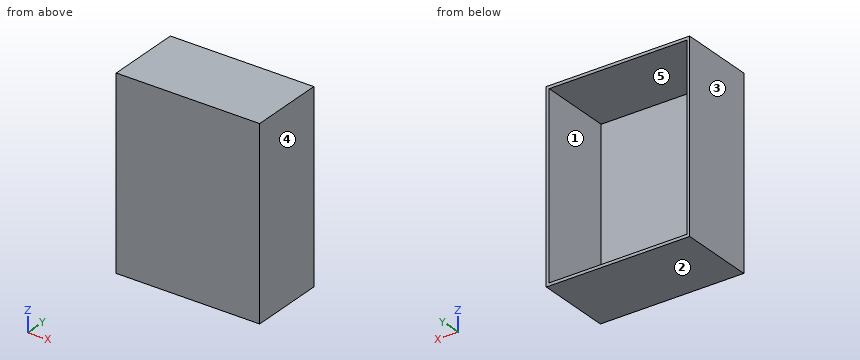
```python
from build123d import *

# Parameters (mm, degrees)
SKETCH2_W   = 99
SKETCH2_H   = 129
SKETCH2_W_2 = 95
SKETCH2_H_2 = 125
WALLS_DEPTH = 50
SKETCH3_W   = 99
SKETCH3_H   = 129
BASE_DEPTH  = 2


with BuildPart() as part:
    # Sketch2 → Walls (new body)
    with BuildSketch(Plane(origin=(0, 0, 0), x_dir=(1, 0, 0), z_dir=(0, 1, 0))):
        Rectangle(SKETCH2_W, SKETCH2_H)
        Rectangle(SKETCH2_W_2, SKETCH2_H_2, mode=Mode.SUBTRACT)
    extrude(amount=WALLS_DEPTH)

    # Sketch3 → Base (add)
    with BuildSketch(Plane.XZ):
        Rectangle(SKETCH3_W, SKETCH3_H)
    extrude(amount=BASE_DEPTH)


solid = part.part
```
The listing builds one solid part. Answer for the finished solid, in the listing's coordinates (mm). Face numbers are marked on the shaded views. A direction names the side the tool comes from. Round coordinates to 2 decimals unless told otherwise and drop trailing zeros. Loops run counter-clockwise (first coordinate to the right, second up) from the corner with the lowest first, then second, coordinate; pieces in that order, holes last. Notation, with made-up numbers: (-8.75, 22.5) - (39.25, 22.5) arc R18 cw to (39.25, 32.5) - close; hole circle Ø4 at (-40, 60.5). An arc over 180 degrees is marked (long way). Return JSON: item names as keys, results as strings. Group by question number.
1. Consider probe 1 along Z at (x, y) = (-37.5, 22); probe 2 along X at (y, z) = (44, -11); probe 3 along Y at (x, z) = (-17, 15). Determine where each line is inside the solid, lowest interval first.
2. The mould has two halves that part along Z. Classify the marked faces 1, 2 and 3: pulls with the +Z half, pulls with the -Z half, needs draft (parallel to the pull), parting line crosses it, or undercut.
3. The part is cut by section C-C on z = 23.5. Determine the outline of the cut face in (x, y).
4. The part is cut by section B-B on x = -19.5. Determine the outline of the cut face in (y, z).
5. The part is cut by section A-A on y = 42. Determine the outline of the cut face in (x, z), then the cut area to 3 significant figures.
6. This flat-tipped pin is pushed along its axis until it touches: P1, Ø10, axis at x = 10, z = 36.5, coming from the +Y side. Where does it stop, or does it pass through?
7. Which of the six approach directions +Z, -Z, +X, -X, +Y, -Y give full straight-line access (tool end or side, diameter ignored) to the marked faces 4 and 5?
Resolved:
{
 "1": {"probe 1": "z = -64.5 to -62.5, 62.5 to 64.5", "probe 2": "x = -49.5 to -47.5, 47.5 to 49.5", "probe 3": "y = -2 to 0"},
 "2": {"face 1": "undercut", "face 2": "pulls with the -Z half", "face 3": "needs draft"},
 "3": {"outline": "(-49.5, -2) - (49.5, -2) - (49.5, 50) - (47.5, 50) - (47.5, 0) - (-47.5, 0) - (-47.5, 50) - (-49.5, 50) - close"},
 "4": {"outline": "(-2, -64.5) - (50, -64.5) - (50, -62.5) - (0, -62.5) - (0, 62.5) - (50, 62.5) - (50, 64.5) - (-2, 64.5) - close"},
 "5": {"outline": "(-49.5, -64.5) - (49.5, -64.5) - (49.5, 64.5) - (-49.5, 64.5) - close; hole (-47.5, -62.5) - (47.5, -62.5) - (47.5, 62.5) - (-47.5, 62.5) - close", "area": "896 mm²"},
 "6": {"P1": "stops at y = 0"},
 "7": {"face 4": "+Z, -Z, +X, +Y, -Y", "face 5": "+Y"}
}
